```python
from build123d import *

# Parameters (mm, degrees)
SKETCH1_R           = 27.5
SKETCH1_R_2         = 11.15
BOSS_EXTRUDE1_DEPTH = 9
CUT_EXTRUDE1_START  = 9
CUT_EXTRUDE1_DEPTH  = 6
CUT_EXTRUDE2_START  = 9
SKETCH3_R           = 39.185897799
SKETCH3_R_2         = 14.15
CUT_EXTRUDE2_DEPTH  = 3.1
CUT_EXTRUDE3_START  = 5.9
SKETCH4_R           = 1.65
CUT_EXTRUDE3_DEPTH  = 6.9
CUT_EXTRUDE9_START  = 9
SKETCH9_R           = 3
CUT_EXTRUDE9_DEPTH  = 3.1
SKETCH8_R           = 3.3
CUT_EXTRUDE10_DEPTH = 2.1


with BuildPart() as part:
    # Sketch1 → Boss-Extrude1 (new body)
    with BuildSketch(Plane.XY):
        Circle(SKETCH1_R)
        Circle(SKETCH1_R_2, mode=Mode.SUBTRACT)
    extrude(amount=BOSS_EXTRUDE1_DEPTH)

    # Sketch2 → Cut-Extrude1 (cut)
    with BuildSketch(Plane.XY.offset(CUT_EXTRUDE1_START)):
        with BuildLine():
            Line((-27.447404249, 1.7), (-24.84017663, 1.7))
            ThreePointArc((-24.84017663, 1.7), (0, 24.898280563), (24.84017663, 1.7))
            Line((24.84017663, 1.7), (27.447404249, 1.7))
            ThreePointArc((27.447404249, 1.7), (0, 27.5), (-27.447404249, 1.7))
        make_face()
        with BuildLine():
            Line((27.447404249, -1.7), (24.841900088, -1.7))
            ThreePointArc((24.841900088, -1.7), (0, -24.9), (-24.841900088, -1.7))
            Line((-24.841900088, -1.7), (-27.447404249, -1.7))
            ThreePointArc((-27.447404249, -1.7), (0, -27.5), (27.447404249, -1.7))
        make_face()
    extrude(amount=-CUT_EXTRUDE1_DEPTH, mode=Mode.SUBTRACT)

    # Sketch3 → Cut-Extrude2 (cut)
    with BuildSketch(Plane.XY.offset(CUT_EXTRUDE2_START)):
        Circle(SKETCH3_R)
        Circle(SKETCH3_R_2, mode=Mode.SUBTRACT)
    extrude(amount=-CUT_EXTRUDE2_DEPTH, mode=Mode.SUBTRACT)

    # Sketch4 → Cut-Extrude3 (cut, through all)
    with BuildSketch(Plane.XY.offset(CUT_EXTRUDE3_START)):
        with Locations((-16.454482672, 9.5)):
            Circle(SKETCH4_R)
        with Locations((16.454482672, 9.5)):
            Circle(SKETCH4_R)
        with Locations((16.454482672, -9.5)):
            Circle(SKETCH4_R)
        with Locations((-16.454482672, -9.5)):
            Circle(SKETCH4_R)
    extrude(amount=-CUT_EXTRUDE3_DEPTH, mode=Mode.SUBTRACT)

    # Sketch9 → Cut-Extrude9 (cut)
    with BuildSketch(Plane.XY.offset(CUT_EXTRUDE9_START)):
        with Locations((-8.530989978, 8.530989978)):
            Circle(SKETCH9_R)
        with Locations((8.530989978, 8.530989978)):
            Circle(SKETCH9_R)
        with Locations((8.530989978, -8.530989978)):
            Circle(SKETCH9_R)
        with Locations((-8.530989978, -8.530989978)):
            Circle(SKETCH9_R)
    extrude(amount=-CUT_EXTRUDE9_DEPTH, mode=Mode.SUBTRACT)

    # Sketch8 → Cut-Extrude10 (cut)
    with BuildSketch(Plane.XY):
        with Locations((-16.454482672, 9.5)):
            Circle(SKETCH8_R)
        with Locations((-16.454482672, -9.5)):
            Circle(SKETCH8_R)
        with Locations((16.454482672, -9.5)):
            Circle(SKETCH8_R)
        with Locations((16.454482672, 9.5)):
            Circle(SKETCH8_R)
    extrude(amount=CUT_EXTRUDE10_DEPTH, mode=Mode.SUBTRACT)


solid = part.part
```
Can you work these out from the model? Positions are in its coordinate system, mm. A direction names the side the tool comes from. Coordinates: 2 decimals unless noted, no trailing zeros. Loops run counter-clockwise (first coordinate to the right, second up) from the corner with the lowest first, then second, coordinate; pieces in that order, holes last.
Item 1: Suppose I cut it at A-A (z = 7). Please give me the cut outline in (x, y).
Answers below:
outline: (-11.52, -8.22) arc R3 cw to (-9.57, -5.72) arc R11.15 cw to (-9.57, 5.72) arc R3 cw to (-11.52, 8.22) arc R14.15 ccw to start; (-8.22, -11.52) arc R14.15 ccw to (8.22, -11.52) arc R3 cw to (5.72, -9.57) arc R11.15 cw to (-5.72, -9.57) arc R3 cw to start; (-8.22, 11.52) arc R3 cw to (-5.72, 9.57) arc R11.15 cw to (5.72, 9.57) arc R3 cw to (8.22, 11.52) arc R14.15 ccw to start; (9.57, -5.72) arc R3 cw to (11.52, -8.22) arc R14.15 ccw to (11.52, 8.22) arc R3 cw to (9.57, 5.72) arc R11.15 cw to start
Item 2: Suppose I cut it at D-D (x = -15.5). Please give me the cut outline in (y, z).
Answers below:
outline: (-22.72, 0) - (-12.66, 0) - (-12.66, 2.1) - (-10.85, 2.1) - (-10.85, 5.9) - (-19.49, 5.9) - (-19.49, 3) - (-22.72, 3) - close; (-8.15, 2.1) - (-6.34, 2.1) - (-6.34, 0) - (6.34, 0) - (6.34, 2.1) - (8.15, 2.1) - (8.15, 5.9) - (-8.15, 5.9) - close; (10.85, 2.1) - (12.66, 2.1) - (12.66, 0) - (22.72, 0) - (22.72, 3) - (19.49, 3) - (19.49, 5.9) - (10.85, 5.9) - close
Item 3: Suppose I cut it at B-B (y = 0). Please give me the cut outline in (x, z).
Answers below:
outline: (-27.5, 0) - (-11.15, 0) - (-11.15, 9) - (-14.15, 9) - (-14.15, 5.9) - (-27.5, 5.9) - close; (11.15, 0) - (27.5, 0) - (27.5, 5.9) - (14.15, 5.9) - (14.15, 9) - (11.15, 9) - close
Item 4: Please list where these lines run through material, in increasing order: L1, parallel to Y at x = 0, z = 4.5; L2, parallel to X at y = -0.5, z = 6.5; L3, parallel to X at y = -9, z = 2.25.
Answers below:
L1: y = -24.9 to -11.15, 11.15 to 24.9
L2: x = -14.14 to -11.14, 11.14 to 14.14
L3: x = -25.99 to -18.03, -14.88 to -6.58, 6.58 to 14.88, 18.03 to 25.99
Item 5: Suppose I cut it at C-C (x = 0). Please give me the cut outline in (y, z).
Answers below:
outline: (-27.5, 0) - (-11.15, 0) - (-11.15, 9) - (-14.15, 9) - (-14.15, 5.9) - (-24.9, 5.9) - (-24.9, 3) - (-27.5, 3) - close; (11.15, 0) - (27.5, 0) - (27.5, 3) - (24.9, 3) - (24.9, 5.9) - (14.15, 5.9) - (14.15, 9) - (11.15, 9) - close
Item 6: I'm going to push flat-ended pins straight in: pin 1 (5.5 mm diameter, centred on x = -16.45, y = -9.5, fed in from -Z); pin 2 (7.5 mm diameter, centred on x = 15, y = -8, fed in from -Z); pin 3 (3 mm diameter, centred on x = 10, z = 1, fed in from +Y); pin 4 (1 mm diameter, centred on x = 18, y = -19, fed in from +Z). Where does each tip first touch, or does it pass through?
Answers below:
pin 1: stops at z = 2.1
pin 2: stops at z = 0
pin 3: stops at y = 26.15
pin 4: stops at z = 3
Item 7: Which directions (+Z, -Z, +X, -X, +Y, -Y) give clear straight access to the entire face, cutting with the end or side of a thin tool? Please do faces 1 (the face through (10.887, 6.674, 7.472)), 2 (the face through (12, -11, 5.9)), 3 (the face through (-0.12, -14.15, 7.47)), 4 (the face through (26, 1.7, 4)).
Answers below:
face 1: +Z, +Y
face 2: +Z
face 3: +Z, -Y
face 4: +Z, +X, +Y
